Check sheet for the modelled part. Datum: model origin and axes. Units: mm. A direction names the side the tool comes from. Round coordinates to 2 decimals unless told otherwise and drop trailing zeros. Order: outer loops, then holes, each group sorted by start corner. A loop starts at its lowest first (then second) coordinate and runs counter-clockwise, first axis right, second up. Notation, with made-up numbers: (-33.75, 82) -> (20.25, 82) arc R11 cw to (20.25, 97) -> close; hole circle Ø6 at (7, 58.25). An arc over 180 degrees is marked (long way). Answer in a Markdown table with one row per item. Add a question column.
1. Sectioned sample at D-D, the plane x = -9.25. Record the boundary of the cut face in (y, z).
2. Access from +Z, -Z, +X, -X, +Y, -Y to the whole of each face (thin tool, end or side, straight path). Record for faces 1 (the flat face through (-12.7, -8.2, -8.2)), 2 (the cylindrical face through (-18.977, -60.267, 2.652)).
3. Depth check by flat-ended pin: P1, Ø5, axis at x = -13, z = 11, coming from the -Y side; P2, Ø8, axis at x = -12.5, y = -31, coming from the -Z side; P3, Ø13.5, axis at y = 0, z = 0, coming from the +X side; P4, Ø10, axis at y = 2, z = -12.5, coming from the -X side. Enter the tip coordinate at first touch or a pass-through.
4. Sectioned sample at A-A, the plane z = 0. Record the boundary of the cut face in (x, y) (3 decimals).
5. Material ranges on L1, parallel to Z at x = -17.25, y = 0 (3 decimals); L2, parallel to Y at x = -6, z = 10; L3, parallel to Z at x = -18.5, y = 17, recorded low to high. Write a range as from..to.
6. Sectioned sample at C-C, the plane x = -17.25. Record the boundary of the cut face in (y, z) (3 decimals).
7. Draft check along Y on faces 3 (the conical face through (-0.672, 52.336, 16.481)), 4 (the flat face through (-25.4, -14, 14)), 5 (the cylindrical face through (-6.26, 10.78, 3.4)). Enter one of: +Y half, -Y half, draft (parallel to the pull), parting line (faces both ways), or undercut.
```python
from build123d import *

# Parameters (mm, degrees)
F0_R           = 60.325
F1_DEPTH       = 25.4
F2_SIZE        = 1.143
F4_D           = 22.606
F4_CBORE_D     = 38.1
F4_CBORE_DEPTH = 12.7


# Not quite as in the source:
# - a fillet or chamfer that OpenCascade refuses, or shapes differently, is made with other operations: its cross-section is extruded or revolved along the edge and cut away or added


with BuildPart() as f1:
    # F0 (on Right) → F1 (new body)
    with BuildSketch(Plane.YZ):
        Circle(F0_R)
    extrude(amount=-F1_DEPTH)

    # F2
    f2_edges = [f1.edges().sort_by_distance(p)[0] for p in [
        (-25.4, -60.325, 0),
        (-12.7, 60.325, 0),
        (0, -60.325, 0),
    ]]
    chamfer(f2_edges, length=F2_SIZE)

    # F4 (through all)
    with Locations(Plane(origin=(-25.4, 0, 0), x_dir=(0, -1, 0), z_dir=(-1, 0, 0))):
        with Locations((0, 0)):
            CounterBoreHole(F4_D / 2, F4_CBORE_D / 2, F4_CBORE_DEPTH)

    # F5: chamfer of 12.7 on 1 edges, made by hand

    # F5_s1 → F5_t2 (revolve, cut)
    with BuildSketch(Plane.XY):
        Polygon((-13.843, 60.325), (7.8372561211, 51.3447438789), (-1.143, 60.325), align=None)
    revolve(axis=Axis((-1.143, 0, 0), (1, 0, 0)), mode=Mode.SUBTRACT)


solid = f1.part
```
Answer key:
| question | item | result |
|---|---|---|
| 1 | outline | circle Ø116.85 at (0, 0); hole circle Ø22.61 at (0, 0) |
| 2 | face 1 | -X |
| 2 | face 2 | +X, -X |
| 3 | P1 | stops at y = -59.7 |
| 3 | P2 | stops at z = -53.83 |
| 3 | P3 | passes through |
| 3 | P4 | stops at x = -12.7 |
| 4 | outline | (-25.4, -59.182) -> (-24.257, -60.325) -> (-13.843, -60.325) -> (0, -54.591) -> (0, -11.303) -> (-12.7, -11.303) -> (-12.7, -19.05) -> (-25.4, -19.05) -> close; (-25.4, 19.05) -> (-12.7, 19.05) -> (-12.7, 11.303) -> (0, 11.303) -> (0, 54.591) -> (-13.843, 60.325) -> (-24.257, 60.325) -> (-25.4, 59.182) -> close |
| 5 | L1 | z = -60.325..-19.05, 19.05..60.325 |
| 5 | L2 | y = -56.19..-5.27, 5.27..56.19 |
| 5 | L3 | z = -57.88..-8.6, 8.6..57.88 |
| 6 | outline | circle Ø120.65 at (0, 0); hole circle Ø38.1 at (0, 0) |
| 7 | face 3 | parting line |
| 7 | face 4 | draft |
| 7 | face 5 | undercut |
